Geometry check sheet. Reference: the model listing, model coordinates, mm. A direction names the side the tool comes from. Round coordinates to 2 decimals unless told otherwise and drop trailing zeros. Write each loop counter-clockwise with the first axis right and the second up, starting at its lowest first coordinate (ties: lowest second). Pieces come first, ordered by that corner, then holes. Notation, with made-up numbers: M 5,27 L 41,27 A12 ccw 41,49 Z; hole C 46.25,48 d1. An arc over 180 degrees is marked long. Answer in a Markdown table with one row per item. Add a question column.
from build123d import *

# Parameters (mm, degrees)
F1_DEPTH = 210.7
F0_W     = 79
F0_H     = 26.5
F0_R     = 3
F2_DEPTH = 2
F3_DEPTH = 2
F4_R     = 1.5
F5_DEPTH = 3
F6_W     = 5
F6_H     = 5
F6_R     = 1.25
F7_DEPTH = 26.5


with BuildPart() as f1:
    # F0 (on Right) → F1 (new body)
    with BuildSketch(Plane.YZ):
        with BuildLine():
            Line((-79, -29.7321164519), (-79, -3.2321164519))
            Line((-79, -3.2321164519), (-82.5, -3.2321164519))
            Line((-82.5, -3.2321164519), (-82.5, -16.2321164519))
            Line((-82.5, -16.2321164519), (-80, -16.2321164519))
            Line((-80, -16.2321164519), (-80, -21.2321164519))
            Line((-80, -21.2321164519), (-82.5, -20.2321164519))
            Line((-82.5, -20.2321164519), (-82.5, -28.2321164519))
            ThreePointArc((-82.5, -28.2321164519), (-81.0355339059, -31.7676503579), (-77.5, -33.2321164519))
            Line((-77.5, -33.2321164519), (-1.5, -33.2321164519))
            ThreePointArc((-1.5, -33.2321164519), (2.0355339059, -31.7676503579), (3.5, -28.2321164519))
            Line((3.5, -28.2321164519), (3.5, -20.2321164519))
            Line((3.5, -20.2321164519), (1, -21.2321164519))
            Line((1, -21.2321164519), (1, -16.2321164519))
            Line((1, -16.2321164519), (3.5, -16.2321164519))
            Line((3.5, -16.2321164519), (3.5, -3.2321164519))
            Line((3.5, -3.2321164519), (0, -3.2321164519))
            Line((0, -3.2321164519), (0, -29.7321164519))
            Line((0, -29.7321164519), (-79, -29.7321164519))
        make_face()
    extrude(amount=-F1_DEPTH)

    # F0 (on Right) → F2 (join)
    with BuildSketch(Plane.YZ):
        with Locations((-39.5, -16.4821164519)):
            Rectangle(F0_W, F0_H)
        with Locations((-68, -9.7321164519)):
            Circle(F0_R, mode=Mode.SUBTRACT)
        Polygon((-80, -16.2321164519), (-82.5, -16.2321164519), (-82.5, -20.2321164519), (-80, -21.2321164519), align=None)
        Polygon((3.5, -20.2321164519), (3.5, -16.2321164519), (1, -16.2321164519), (1, -21.2321164519), align=None)
    extrude(amount=F2_DEPTH)

    # F0 (on Right) → F3 (join, through all)
    with BuildSketch(Plane.YZ):
        with BuildLine():
            Line((-79, -29.7321164519), (-79, -3.2321164519))
            Line((-79, -3.2321164519), (-82.5, -3.2321164519))
            Line((-82.5, -3.2321164519), (-82.5, -16.2321164519))
            Line((-82.5, -16.2321164519), (-80, -16.2321164519))
            Line((-80, -16.2321164519), (-80, -21.2321164519))
            Line((-80, -21.2321164519), (-82.5, -20.2321164519))
            Line((-82.5, -20.2321164519), (-82.5, -28.2321164519))
            ThreePointArc((-82.5, -28.2321164519), (-81.0355339059, -31.7676503579), (-77.5, -33.2321164519))
            Line((-77.5, -33.2321164519), (-1.5, -33.2321164519))
            ThreePointArc((-1.5, -33.2321164519), (2.0355339059, -31.7676503579), (3.5, -28.2321164519))
            Line((3.5, -28.2321164519), (3.5, -20.2321164519))
            Line((3.5, -20.2321164519), (1, -21.2321164519))
            Line((1, -21.2321164519), (1, -16.2321164519))
            Line((1, -16.2321164519), (3.5, -16.2321164519))
            Line((3.5, -16.2321164519), (3.5, -3.2321164519))
            Line((3.5, -3.2321164519), (0, -3.2321164519))
            Line((0, -3.2321164519), (0, -29.7321164519))
            Line((0, -29.7321164519), (-79, -29.7321164519))
        make_face()
    extrude(amount=F3_DEPTH)

    # F4 (on face) → F5 (join)
    with BuildSketch(Plane(origin=(-210.7, 0, 0), x_dir=(0, -1, 0), z_dir=(-1, 0, 0))):
        with BuildLine():
            Line((39.8976451881, -3.2321164519), (0, -3.2321164519))
            Line((0, -3.2321164519), (0, -29.7321164519))
            Line((0, -29.7321164519), (79, -29.7321164519))
            Line((79, -29.7321164519), (79, -3.2321164519))
            Line((79, -3.2321164519), (42.5981824726, -3.2321164519))
            ThreePointArc((42.5981824726, -3.2321164519), (42.7783306428, -3.6368593662), (42.839971074, -4.0755741336))
            ThreePointArc((42.839971074, -4.0755741336), (40.809199063, -5.605990946), (39.8976451881, -3.2321164519))
        make_face()
        with Locations((17.6456464854, -19.2755741336)):
            Circle(F4_R, mode=Mode.SUBTRACT)
        with BuildLine():
            Line((20.5, -21.1070965323), (21.4456464854, -16.2070965323))
            ThreePointArc((21.4456464854, -16.2070965323), (22.4815067005, -14.4619803054), (24.3912929708, -13.7755741336))
            Line((24.3912929708, -13.7755741336), (57.8, -13.7755741336))
            ThreePointArc((57.8, -13.7755741336), (59.7097862703, -14.4619803054), (60.7456464854, -16.2070965323))
            Line((60.7456464854, -16.2070965323), (61.6912929708, -21.1070965323))
            ThreePointArc((61.6912929708, -21.1070965323), (61.0592403136, -23.5853604038), (58.7456464854, -24.6755741336))
            Line((58.7456464854, -24.6755741336), (23.4456464854, -24.6755741336))
            ThreePointArc((23.4456464854, -24.6755741336), (21.1320526572, -23.5853604038), (20.5, -21.1070965323))
        make_face(mode=Mode.SUBTRACT)
        with Locations((64.5456464854, -19.2755741336)):
            Circle(F4_R, mode=Mode.SUBTRACT)
        with BuildLine():
            Line((0, -3.2321164519), (-3.5, -3.2321164519))
            Line((-3.5, -3.2321164519), (-3.5, -16.2321164519))
            Line((-3.5, -16.2321164519), (-1, -16.2321164519))
            Line((-1, -16.2321164519), (-1, -21.2321164519))
            Line((-1, -21.2321164519), (-3.5, -20.2321164519))
            Line((-3.5, -20.2321164519), (-3.5, -28.2321164519))
            ThreePointArc((-3.5, -28.2321164519), (-2.0355339059, -31.7676503579), (1.5, -33.2321164519))
            Line((1.5, -33.2321164519), (77.5, -33.2321164519))
            ThreePointArc((77.5, -33.2321164519), (81.0355339059, -31.7676503579), (82.5, -28.2321164519))
            Line((82.5, -28.2321164519), (82.5, -20.2321164519))
            Line((82.5, -20.2321164519), (80, -21.2321164519))
            Line((80, -21.2321164519), (80, -16.2321164519))
            Line((80, -16.2321164519), (82.5, -16.2321164519))
            Line((82.5, -16.2321164519), (82.5, -3.2321164519))
            Line((82.5, -3.2321164519), (79, -3.2321164519))
            Line((79, -3.2321164519), (79, -29.7321164519))
            Line((79, -29.7321164519), (0, -29.7321164519))
            Line((0, -29.7321164519), (0, -3.2321164519))
        make_face()
    extrude(amount=F5_DEPTH)

    # F6 (on face) → F7 (join, through all)
    with BuildSketch(Plane.XY.offset(-29.7321164519)):
        with Locations((-2.5, -76.5)):
            Rectangle(F6_W, F6_H)
        with Locations((-2.5, -76.6462582126)):
            Circle(F6_R, mode=Mode.SUBTRACT)
        with Locations((-2.5, -2.5)):
            Rectangle(F6_W, F6_H)
        with Locations((-2.5, -2.3537417874)):
            Circle(F6_R, mode=Mode.SUBTRACT)
        with Locations((-208.2, -2.5)):
            Rectangle(F6_W, F6_H)
        with Locations((-208.2, -2.3537417874)):
            Circle(F6_R, mode=Mode.SUBTRACT)
        with Locations((-208.2, -76.5)):
            Rectangle(F6_W, F6_H)
        with Locations((-208.2, -76.6462582126)):
            Circle(F6_R, mode=Mode.SUBTRACT)
    extrude(amount=F7_DEPTH)


solid = f1.part
Item 1: Scan lines: probe 1 along Y at (x, z) = (-103, -9.5); probe 2 along X at (y, z) = (-32, -6.25); probe 3 along X at (y, z) = (-4.5, -24.5). Record each from-to range of solid material in increasing order. Write a range as from..to.
Item 2: Section check B-B, the plane y = -13.5. Record the boundary of the cut face in (x, z).
Item 3: Section check C-C, the plane x = -156.5. Record the boundary of the cut face in (y, z), and give its area (3 significant figures).
Item 4: Section check D-D, the plane y = -55.5. Record the boundary of the cut face in (x, z).
Item 5: Gauge pin test, flat ends, axial feed: pin 1 Ø3 at (x, y) = (-208.5, -76) entering from +Z; pin 2 Ø1.5 at (x, z) = (-157, -19) entering from -Y; pin 3 Ø1 at (x, z) = (-165, -18.5) entering from +Y; pin 4 Ø6 at (x, y) = (-186.5, -15.5) entering from +Z. Record the tip position at first contact, or that the pin passes through.
Item 6: Mould release check, pull along X, two halves, no side actions. Record for faces 4 (the flat face through (-104, -79, -17)), 5 (the flat face through (2, -40, -18)), 6 (the flat face through (-213.7, -39, -25)): +X half, -X half, draft (parallel to the pull), parting line (faces both ways), or undercut.
Item 7: Access from +Z, -Z, +X, -X, +Y, -Y to the whole of each face (thin tool, end or side, straight path). Record for faces 1 (the cylindrical face through (0.99, -70.38, -11.56)), 2 (the flat face through (-106, 2, -3.232)), 3 (the flat face through (-5, -77, -17)).
Item 8: Section check A-A, the plane y = -68. Record the boundary of the cut face in (x, z), and give its area (3 significant figures).
Result sheet:
| question | item | result |
|---|---|---|
| 1 | probe 1 | y = -82.5..-79, 0..3.5 |
| 1 | probe 2 | x = -213.7..-210.7, 0..2 |
| 1 | probe 3 | x = -213.7..-205.7, -5..2 |
| 2 | outline | M -213.7,-33.23 L 2,-33.23 L 2,-3.23 L 0,-3.23 L 0,-29.73 L -210.7,-29.73 L -210.7,-3.23 L -213.7,-3.23 Z |
| 3 | outline | M -82.5,-28.23 A5 ccw -77.5,-33.23 L -1.5,-33.23 A5 ccw 3.5,-28.23 L 3.5,-20.23 L 1,-21.23 L 1,-16.23 L 3.5,-16.23 L 3.5,-3.23 L 0,-3.23 L 0,-29.73 L -79,-29.73 L -79,-3.23 L -82.5,-3.23 L -82.5,-16.23 L -80,-16.23 L -80,-21.23 L -82.5,-20.23 Z |
| 3 | area | 453 mm^2 |
| 4 | outline | M -213.7,-33.23 L 2,-33.23 L 2,-3.23 L 0,-3.23 L 0,-29.73 L -210.7,-29.73 L -210.7,-24.68 L -213.7,-24.68 Z; M -213.7,-13.78 L -210.7,-13.78 L -210.7,-3.23 L -213.7,-3.23 Z |
| 5 | pin 1 | stops at z = -3.23 |
| 5 | pin 2 | stops at y = -80 |
| 5 | pin 3 | stops at y = 1 |
| 5 | pin 4 | stops at z = -29.73 |
| 6 | face 4 | undercut |
| 6 | face 5 | +X half |
| 6 | face 6 | -X half |
| 7 | face 1 | +X |
| 7 | face 2 | +Z, +X, -X, +Y, -Y |
| 7 | face 3 | +Z |
| 8 | outline | M -213.7,-33.23 L 2,-33.23 L 2,-12.73 L 0,-12.73 L 0,-29.73 L -210.7,-29.73 L -210.7,-3.23 L -213.7,-3.23 Z; M 0,-6.73 L 2,-6.73 L 2,-3.23 L 0,-3.23 Z |
| 8 | area | 875 mm^2 |
